Geometry check sheet. Reference: the model listing, model coordinates, mm. A direction names the side the tool comes from. Coordinates: 2 decimals unless noted, no trailing zeros. Answer in a Markdown table with one row per item. Add a question column.
1. Mould release check, pull along Y, two halves, no side actions. Record for faces 3 (the flat face through (7, -6.967, 5)), 4 (the flat face through (8, 0, 8.273)), 5 (the flat face through (7, 36, 10)): pulls with the +Y half, pulls with the -Y half, needs draft (parallel to the pull), parting line crosses it, or undercut.
2. Set-up check for faces 1 (the flat face through (148.004, 34.9, 3.8)), 2 (the flat face through (-117, 0, 8.273)): record each of +Z, -Z, +X, -X, +Y, -Y from which the full face is reachable in a straight line by a thin tool's end or side.
3. Depth check by flat-ended pin: P1, Ø4.5, axis at x = -116.5, y = -1.97, coming from the -Z side; P2, Ø3, axis at x = 133.5, y = -1.97, coming from the +Z side; P3, Ø3.5, axis at x = 9.5, y = -1.5, coming from the +Z side. Enter the tip coordinate at first touch or a pass-through.
4. Scan lines: L1, parallel to X at y = 72, z = 5; L2, parallel to Y at x = -126.25, z = 5. Record each from-to range of solid material in increasing order. Write a range as from..to.
```python
from build123d import *

# Parameters (mm, degrees)
SKETCH1_W                                           = 279
SKETCH1_H                                           = 85
BOSS_EXTRUDE1_DEPTH                                 = 10
CBORE_FOR_4_BINDING_HEAD_MACHINE_SCREW1_D           = 3.4544
CBORE_FOR_4_BINDING_HEAD_MACHINE_SCREW1_CBORE_D     = 6.74624
CBORE_FOR_4_BINDING_HEAD_MACHINE_SCREW1_CBORE_DEPTH = 1.7272
F_4_40_TAPPED_HOLE1_D                               = 2.2606
F_4_40_TAPPED_HOLE1_DEPTH                           = 7.6
F_4_40_TAPPED_HOLE1_TIP                             = 0.679152758
F_4_40_TAPPED_HOLE2_D                               = 2.2606
F_4_40_TAPPED_HOLE2_DEPTH                           = 7.6
F_4_40_TAPPED_HOLE2_TIP                             = 0.679152758
F_4_40_TAPPED_HOLE3_D                               = 2.2606
F_4_40_TAPPED_HOLE3_DEPTH                           = 7.6
F_4_40_TAPPED_HOLE3_TIP                             = 0.679152758


with BuildPart() as part:
    # Sketch1 → Boss-Extrude1 (new body)
    with BuildSketch(Plane.XY):
        with Locations((8.503783102, 35.532786885)):
            Rectangle(SKETCH1_W, SKETCH1_H)
    extrude(amount=BOSS_EXTRUDE1_DEPTH)

    # CBORE for #4 Binding Head Machine Screw1 (through all)
    with Locations(Plane.XY.offset(10)):
        with Locations((-116.496216898, -1.967213115), (8.503783102, -1.967213115), (133.503783102, -1.967213115)):
            CounterBoreHole(CBORE_FOR_4_BINDING_HEAD_MACHINE_SCREW1_D / 2, CBORE_FOR_4_BINDING_HEAD_MACHINE_SCREW1_CBORE_D / 2, CBORE_FOR_4_BINDING_HEAD_MACHINE_SCREW1_CBORE_DEPTH)

    # #4-40 Tapped Hole1
    with Locations(Plane.ZY.offset(130.996216898)):
        with Locations((5, 63.032786885), (5, 35.532786885), (5, 8.032786885)):
            Hole(F_4_40_TAPPED_HOLE1_D / 2, depth=F_4_40_TAPPED_HOLE1_DEPTH)
            with Locations((0, 0, -(F_4_40_TAPPED_HOLE1_DEPTH + F_4_40_TAPPED_HOLE1_TIP / 2))):  # 118° drill point
                Cone(0, F_4_40_TAPPED_HOLE1_D / 2, F_4_40_TAPPED_HOLE1_TIP, mode=Mode.SUBTRACT)

    # #4-40 Tapped Hole2
    with Locations(Plane(origin=(148.003783102, 0, 0), x_dir=(0, 0, -1), z_dir=(1, 0, 0))):
        with Locations((-5, 63.032786885), (-5, 35.532786885), (-5, 8.032786885)):
            Hole(F_4_40_TAPPED_HOLE2_D / 2, depth=F_4_40_TAPPED_HOLE2_DEPTH)
            with Locations((0, 0, -(F_4_40_TAPPED_HOLE2_DEPTH + F_4_40_TAPPED_HOLE2_TIP / 2))):  # 118° drill point
                Cone(0, F_4_40_TAPPED_HOLE2_D / 2, F_4_40_TAPPED_HOLE2_TIP, mode=Mode.SUBTRACT)

    # #4-40 Tapped Hole3
    with Locations(Plane(origin=(0, 78.032786885, 0), x_dir=(1, 0, 0), z_dir=(0, 1, 0))):
        with Locations((-91.496216898, -5), (108.503783102, -5)):
            Hole(F_4_40_TAPPED_HOLE3_D / 2, depth=F_4_40_TAPPED_HOLE3_DEPTH)
            with Locations((0, 0, -(F_4_40_TAPPED_HOLE3_DEPTH + F_4_40_TAPPED_HOLE3_TIP / 2))):  # 118° drill point
                Cone(0, F_4_40_TAPPED_HOLE3_D / 2, F_4_40_TAPPED_HOLE3_TIP, mode=Mode.SUBTRACT)


solid = part.part
```
Results found:
| question | item | result |
|---|---|---|
| 1 | face 3 | pulls with the -Y half |
| 1 | face 4 | undercut |
| 1 | face 5 | needs draft |
| 2 | face 1 | +Z, -Z, +X, +Y, -Y |
| 2 | face 2 | +Z |
| 3 | P1 | stops at z = 0 |
| 3 | P2 | passes through |
| 3 | P3 | stops at z = 8.27 |
| 4 | L1 | x = -131..-92.63, -90.37..107.37, 109.63..148 |
| 4 | L2 | y = -6.97..6.9, 9.16..34.4, 36.66..61.9, 64.16..78.03 |
